Input: part model. Units: mm. Frame: model coordinates. Face numbers are marked on the shaded views. A direction names the side the tool comes from. Round coordinates to 2 decimals unless told otherwise and drop trailing zeros. Loops run counter-clockwise (first coordinate to the right, second up) from the corner with the lowest first, then second, coordinate; pieces in that order, holes last. Notation, with made-up numbers: (52.5, 61) - (80.5, 61) arc R13 cw to (80.5, 71) - close; hole circle Ø4 at (-20, 18.5). An arc over 180 degrees is marked (long way). Use CSV: the item, a comma, the result in double quotes. Start each with the question number.
1. Pin query (flat end, axial travel): P1, Ø1, axis at y = 12, z = 19, coming from the -X side; P2, Ø2.5, axis at x = -15.5, y = 0, coming from the +Z side; P3, Ø3.5, axis at x = -15, y = 0.5, coming from the +Z side. Return the tip coordinate at first contact, or that it passes through.
2. Cut plane B-B (y = 0). Return loops of the section in (x, z).
3. Cut plane A-A (x = 0). Return loops of the section in (y, z).
4. Cut plane D-D (x = -15.5). Return loops of the section in (y, z), and give its area (3 significant figures).
5. Access query for the marked faces 1, 2 and 3. Directions: +Z, -Z, +X, -X, +Y, -Y. A direction counts if a zero-diameter tool reaches every point of the face in a straight line with its end or side. Return the directions, or none.
6. Material intervals for probe 1 along Z at (x, y) = (11, 8); probe 2 along Z at (x, y) = (12.5, -13.5); probe 3 along Y at (x, z) = (-7.75, 51), sorted ascending. Write a range as from..to.
7. Cut plane C-C (z = 31). Return loops of the section in (x, y).
```python
from build123d import *

# Parameters (mm, degrees)
SKETCH1_R           = 16.5
BOSS_EXTRUDE1_DEPTH = 29
SKETCH2_R           = 18.5
BOSS_EXTRUDE2_DEPTH = 24
SKETCH3_R           = 6
BOSS_EXTRUDE3_DEPTH = 6
SKETCH4_R           = 3
BOSS_EXTRUDE5_DEPTH = 3
BOSS_EXTRUDE6_DEPTH = 12
BOSS_EXTRUDE8_START = 12
SKETCH6_R           = 16.5
BOSS_EXTRUDE8_DEPTH = 12
SKETCH7_R           = 1.5
CUT_EXTRUDE1_DEPTH  = 5


with BuildPart() as part:
    # Sketch1 → Boss-Extrude1 (new body)
    with BuildSketch(Plane.XY):
        with Locations(Location((0, 0, 0), (0, 0, 180))):
            Circle(SKETCH1_R)
    extrude(amount=BOSS_EXTRUDE1_DEPTH)

    # Sketch2 → Boss-Extrude2 (add)
    with BuildSketch(Plane.XY.offset(29)):
        Circle(SKETCH2_R)
    extrude(amount=BOSS_EXTRUDE2_DEPTH)

    # Sketch3 → Boss-Extrude3 (add)
    with BuildSketch(Plane.XY.offset(53)):
        with Locations((0, 7)):
            Circle(SKETCH3_R)
    extrude(amount=BOSS_EXTRUDE3_DEPTH)

    # Sketch4 → Boss-Extrude5 (add)
    with BuildSketch(Plane.XY.offset(59)):
        with Locations((0, 7)):
            Circle(SKETCH4_R)
    extrude(amount=BOSS_EXTRUDE5_DEPTH)

    # Sketch5 → Boss-Extrude6 (add)
    with BuildSketch(Plane.XY.offset(62)):
        with BuildLine():
            Line((-1.658312395, 9.5), (1.658312395, 9.5))
            ThreePointArc((1.658312395, 9.5), (0, 4), (-1.658312395, 9.5))
        make_face()
    extrude(amount=BOSS_EXTRUDE6_DEPTH)

    # Sketch6 → Boss-Extrude8 (add)
    with BuildSketch(Plane(origin=(0, 0, 0), x_dir=(-1, 0, 0), z_dir=(0, 0, -1)).offset(BOSS_EXTRUDE8_START)):
        Circle(SKETCH6_R)
    extrude(amount=-BOSS_EXTRUDE8_DEPTH)

    # Sketch7 → Cut-Extrude1 (cut)
    with BuildSketch(Plane.XY.offset(53)):
        with Locations((-15.5, 0)):
            Circle(SKETCH7_R)
        with Locations((7.75, 13.423393759)):
            Circle(SKETCH7_R)
        with Locations((7.75, -13.423393759)):
            Circle(SKETCH7_R)
        with Locations((15.5, 0)):
            Circle(SKETCH7_R)
        with Locations((-7.75, -13.423393759)):
            Circle(SKETCH7_R)
        with Locations((-7.75, 13.423393759)):
            Circle(SKETCH7_R)
    extrude(amount=-CUT_EXTRUDE1_DEPTH, mode=Mode.SUBTRACT)


solid = part.part
```
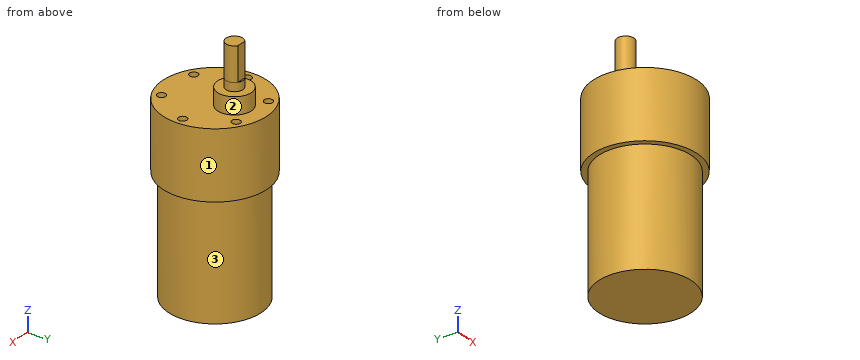
Established:
1,P1,"stops at x = -11.83"
1,P2,"stops at z = 48"
1,P3,"stops at z = 53"
2,outline,"(-18.5, 29) - (-16.5, 29) - (-16.5, -12) - (16.5, -12) - (16.5, 29) - (18.5, 29) - (18.5, 53) - (17, 53) - (17, 48) - (14, 48) - (14, 53) - (-14, 53) - (-14, 48) - (-17, 48) - (-17, 53) - (-18.5, 53) - close"
3,outline,"(-18.5, 29) - (-16.5, 29) - (-16.5, -12) - (16.5, -12) - (16.5, 29) - (18.5, 29) - (18.5, 53) - (13, 53) - (13, 59) - (10, 59) - (10, 62) - (9.5, 62) - (9.5, 74) - (4, 74) - (4, 59) - (1, 59) - (1, 53) - (-18.5, 53) - close"
4,outline,"(-10.1, 29) - (-5.66, 29) - (-5.66, -12) - (5.66, -12) - (5.66, 29) - (10.1, 29) - (10.1, 53) - (1.5, 53) - (1.5, 48) - (-1.5, 48) - (-1.5, 53) - (-10.1, 53) - close"
4,area,"934 mm2"
5,face 1,"+Z, -Z"
5,face 2,"+Z"
5,face 3,"-Z"
6,probe 1,"z = -12..53"
6,probe 2,"z = 29..53"
6,probe 3,"y = -16.8..-14.92, -11.92..11.92, 14.92..16.8"
7,outline,"circle Ø37 at (0, 0)"
